Here's how the part is built. I have some questions about the finished solid (model axes, mm). Coordinates: 2 decimals unless noted, no trailing zeros. Order: outer loops, then holes, each group sorted by start corner. A loop starts at its lowest first (then second) coordinate and runs counter-clockwise, first axis right, second up. Notation, with made-up numbers: (-29, 20) - (22, 20) arc R25 ccw to (22, 32) - close; hole circle Ø11 at (-21, 34). An arc over 180 degrees is marked (long way). Answer in a Markdown table with one row per item. Add a question column.
Item 1: I want a section at D-D (z = -7). Please give me the cut outline in (x, y).
Item 2: I want a section at C-C (y = 0.7). Please give me the cut outline in (x, z), plus the area to 3 significant figures.
Item 3: Will this pin go through, and if not, where does the flat tip stop? pin 1 Ø4 at (x, z) = (19, -26.5) entering from -Y.
Item 4: I want a section at B-B (x = 19). Please give me the cut outline in (y, z), plus the area to 3 significant figures.
Item 5: If I drill on line 1 along Z through (x, y) = (-19, -0.35); line 2 along Z through (x, y) = (7.5, 0.85); line 3 along Z through (x, y) = (-17.5, 0.4), over which ranges is the centre line in solid material (lowest first)? Write a range as from..to.
Item 6: I want a section at A-A (z = -26.5). Please give me the cut outline in (x, y).
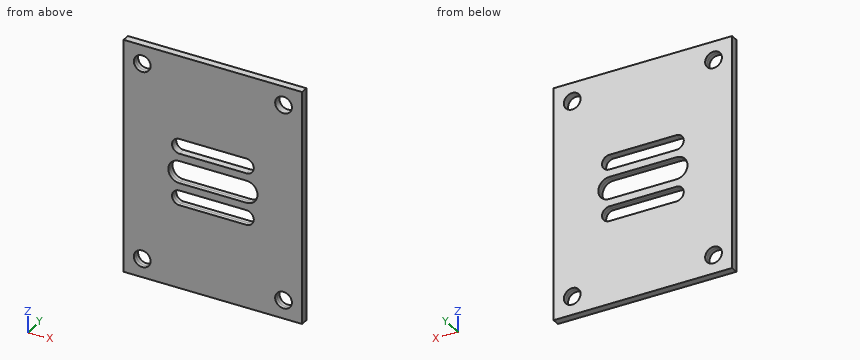
```python
from build123d import *

# Parameters (mm, degrees)
F0_W     = 48
F0_H     = 63
F0_R     = 2.25
F1_DEPTH = 1


with BuildPart() as f1:
    # F0 (on Front) → F1 (new body, symmetric)
    with BuildSketch(Plane.XZ):
        Rectangle(F0_W, F0_H)
        with Locations((-19, -26.5)):
            Circle(F0_R, mode=Mode.SUBTRACT)
        with Locations((19, -26.5)):
            Circle(F0_R, mode=Mode.SUBTRACT)
        with BuildLine():
            Line((9, -9), (-9, -9))
            ThreePointArc((-9, -9), (-11, -7), (-9, -5))
            Line((-9, -5), (9, -5))
            ThreePointArc((9, -5), (11, -7), (9, -9))
        make_face(mode=Mode.SUBTRACT)
        with Locations((-19, 26.5)):
            Circle(F0_R, mode=Mode.SUBTRACT)
        with BuildLine():
            Line((9, -3), (-9, -3))
            ThreePointArc((-9, -3), (-11.1213203436, -2.1213203436), (-12, 0))
            ThreePointArc((-12, 0), (-11.1213203436, 2.1213203436), (-9, 3))
            Line((-9, 3), (0, 3))
            Line((0, 3), (9, 3))
            ThreePointArc((9, 3), (11.1213203436, 2.1213203436), (12, 0))
            ThreePointArc((12, 0), (11.1213203436, -2.1213203436), (9, -3))
        make_face(mode=Mode.SUBTRACT)
        with BuildLine():
            Line((9, 5), (-9, 5))
            ThreePointArc((-9, 5), (-11, 7), (-9, 9))
            Line((-9, 9), (9, 9))
            ThreePointArc((9, 9), (11, 7), (9, 5))
        make_face(mode=Mode.SUBTRACT)
        with Locations((19, 26.5)):
            Circle(F0_R, mode=Mode.SUBTRACT)
    extrude(amount=F1_DEPTH, both=True)


solid = f1.part
```
Values follow:
| question | item | result |
|---|---|---|
| 1 | outline | (-24, -1) - (-11, -1) - (-11, 1) - (-24, 1) - close; (11, -1) - (24, -1) - (24, 1) - (11, 1) - close |
| 2 | outline | (-24, -31.5) - (24, -31.5) - (24, 31.5) - (-24, 31.5) - close; hole circle Ø4.5 at (-19, -26.5); hole circle Ø4.5 at (-19, 26.5); hole (-9, -9) - (9, -9) arc R2 ccw to (9, -5) - (-9, -5) arc R2 ccw to start; hole (-9, -3) - (9, -3) arc R3 ccw to (9, 3) - (-9, 3) arc R3 ccw to start; hole (-9, 5) - (9, 5) arc R2 ccw to (9, 9) - (-9, 9) arc R2 ccw to start; hole circle Ø4.5 at (19, -26.5); hole circle Ø4.5 at (19, 26.5) |
| 2 | area | 2,650 mm^2 |
| 3 | pin 1 | passes through |
| 4 | outline | (-1, -31.5) - (1, -31.5) - (1, -28.75) - (-1, -28.75) - close; (-1, -24.25) - (1, -24.25) - (1, 24.25) - (-1, 24.25) - close; (-1, 28.75) - (1, 28.75) - (1, 31.5) - (-1, 31.5) - close |
| 4 | area | 108 mm^2 |
| 5 | line 1 | z = -31.5..-28.75, -24.25..24.25, 28.75..31.5 |
| 5 | line 2 | z = -31.5..-9, -5..-3, 3..5, 9..31.5 |
| 5 | line 3 | z = -31.5..-28.18, -24.82..24.82, 28.18..31.5 |
| 6 | outline | (-24, -1) - (-21.25, -1) - (-21.25, 1) - (-24, 1) - close; (-16.75, -1) - (16.75, -1) - (16.75, 1) - (-16.75, 1) - close; (21.25, -1) - (24, -1) - (24, 1) - (21.25, 1) - close |
